```python
from build123d import *

# Parameters (mm, degrees)
F0_R     = 2
F0_R_2   = 2.5
F0_W     = 48
F0_H     = 45
F1_DEPTH = 3
F2_W     = 58
F2_H     = 66
F2_W_2   = 54
F2_H_2   = 62
F3_DEPTH = 10
F4_R     = 2
F5_DEPTH = 150
F6_R     = 2
F7_DEPTH = 150


with BuildPart() as f1:
    # F0 (on Top) → F1 (new body)
    with BuildSketch(Plane.XY):
        with BuildLine():
            Line((-29, -33), (29, -33))
            Line((29, -33), (29, -15.492203))
            ThreePointArc((29, -15.492203), (31.928932, -8.421135), (39, -5.492203))
            Line((39, -5.492203), (41.707241, -5.492203))
            ThreePointArc((41.707241, -5.492203), (47.49805, -0.146431), (42, 5.5))
            Line((42, 5.5), (39, 5.5))
            ThreePointArc((39, 5.5), (31.928932, 8.428932), (29, 15.5))
            Line((29, 15.5), (29, 33))
            Line((29, 33), (-29, 33))
            Line((-29, 33), (-29, 15.5))
            ThreePointArc((-29, 15.5), (-31.928932, 8.428932), (-39, 5.5))
            Line((-39, 5.5), (-42, 5.5))
            ThreePointArc((-42, 5.5), (-47.49805, -0.146431), (-41.707241, -5.492203))
            Line((-41.707241, -5.492203), (-39, -5.492203))
            ThreePointArc((-39, -5.492203), (-31.928932, -8.421135), (-29, -15.492203))
            Line((-29, -15.492203), (-29, -33))
        make_face()
        with Locations((0, -27)):
            Circle(F0_R, mode=Mode.SUBTRACT)
        with Locations((-42, 0)):
            Circle(F0_R, mode=Mode.SUBTRACT)
        with Locations((-27, 0)):
            Circle(F0_R_2, mode=Mode.SUBTRACT)
        Rectangle(F0_W, F0_H, mode=Mode.SUBTRACT)
        with Locations((27, 0)):
            Circle(F0_R_2, mode=Mode.SUBTRACT)
        with Locations((42, 0)):
            Circle(F0_R, mode=Mode.SUBTRACT)
        with Locations((0, 27)):
            Circle(F0_R, mode=Mode.SUBTRACT)
    extrude(amount=F1_DEPTH)

    # F2 (on face) → F3 (join)
    with BuildSketch(Plane.XY.offset(3)):
        Rectangle(F2_W, F2_H)
        Rectangle(F2_W_2, F2_H_2, mode=Mode.SUBTRACT)
    extrude(amount=F3_DEPTH)

    # F4 (on face) → F5 (cut)
    with BuildSketch(Plane.XZ.offset(33)):
        with Locations((-15, 6.5)):
            Circle(F4_R)
        with Locations((15, 6.5)):
            Circle(F4_R)
    extrude(amount=-F5_DEPTH, mode=Mode.SUBTRACT)

    # F6 (on face) → F7 (cut)
    with BuildSketch(Plane.YZ.offset(29)):
        with Locations((-16, 6.5)):
            Circle(F6_R)
        with Locations((16, 6.5)):
            Circle(F6_R)
    extrude(amount=-F7_DEPTH, mode=Mode.SUBTRACT)


solid = f1.part
```
The model under review builds one solid part; all positions refer to its coordinate system, in mm. A direction names the side the tool comes from. Round coordinates to 2 decimals unless told otherwise and drop trailing zeros. Write each loop counter-clockwise with the first axis right and the second up, starting at its lowest first coordinate (ties: lowest second). Pieces come first, ordered by that corner, then holes.
(1) Insertion check: pin 1 (0.9 mm diameter, centred on y = 4.5, z = 1.5, fed in from -X); pin 2 (2 mm diameter, centred on y = -8.5, z = 4.5, fed in from +X); pin 3 (0.6 mm diameter, centred on x = 28, y = -0.5, fed in from -Z). Each pin has a flat end and moves straight along its axis. Give the tip position at first contact, or say it passes through.
(2) Machinability: for faces 1 (the flat face through (41, 5.5, 1)), 2 (the flat face through (0, -31, 8)), 3 (the flat face through (36, 0, 3)), 4 (the flat face through (-28, 0, 3)), which of the approach directions +Z, -Z, +X, -X, +Y, -Y give a long, thin tool a straight path to every point of the face, cutting with its end or side? Answer none if there is none.
(3) Mouldability with a two-part tool opening along X and no side actions: class faces 5 (the flat face through (0, -33, 6)), 6 (the flat face through (-27, 0, 8)), 7 (the flat face through (0, 22.5, 1)), 8 (the cylindrical face through (-31.85, 8.51, 1.48)) as +X half, -X half, draft (parallel to the pull), parting line (faces both ways), or undercut.
(4) We need section B-B on x = 15. Give the boundary of the cut face in (y, z), and give its area (3 significant figures).
(5) We need section A-A on y = -27. Give the boundary of the cut face in (x, z).
(6) Wall thickness on L1, parallel to Z at x = 27.85, y = -16; L2, parallel to X at y = -20.5, z = 4.5; L3, parallel to Y at x = 7, z = 6.75: over which ranges is each line inside the solid? List them lowest first.
(7) We need section D-D on x = 36. Give the boundary of the cut face in (y, z), and give its area (3 significant figures).
(8) We need section C-C on y = 6.5. Give the boundary of the cut face in (x, z).
Findings below:
1. pin 1: stops at x = -45.72
1. pin 2: stops at x = 29
1. pin 3: stops at z = 3
2. face 1: +Z, -Z, +X, +Y
2. face 2: +Z
2. face 3: +Z, +X, +Y, -Y
2. face 4: -Z
3. face 5: draft
3. face 6: undercut
3. face 7: undercut
3. face 8: -X half
4. outline: (-33, 0) - (-22.5, 0) - (-22.5, 3) - (-31, 3) - (-31, 4.5) - (-33, 4.5) - close; (-33, 8.5) - (-31, 8.5) - (-31, 13) - (-33, 13) - close; (22.5, 0) - (33, 0) - (33, 4.5) - (31, 4.5) - (31, 3) - (22.5, 3) - close; (31, 8.5) - (33, 8.5) - (33, 13) - (31, 13) - close
4. area: 87.0 mm2
5. outline: (-29, 0) - (-2, 0) - (-2, 3) - (-27, 3) - (-27, 13) - (-29, 13) - close; (2, 0) - (29, 0) - (29, 13) - (27, 13) - (27, 3) - (2, 3) - close
6. L1: z = 0 to 4.5, 8.5 to 13
6. L2: x = -29 to -27, 27 to 29
6. L3: y = -33 to -31, 31 to 33
7. outline: (-5.95, 0) - (5.96, 0) - (5.96, 3) - (-5.95, 3) - close
7. area: 35.7 mm2
8. outline: (-34.64, 0) - (-24, 0) - (-24, 3) - (-27, 3) - (-27, 13) - (-29, 13) - (-29, 3) - (-34.64, 3) - close; (24, 0) - (34.64, 0) - (34.64, 3) - (29, 3) - (29, 13) - (27, 13) - (27, 3) - (24, 3) - close
